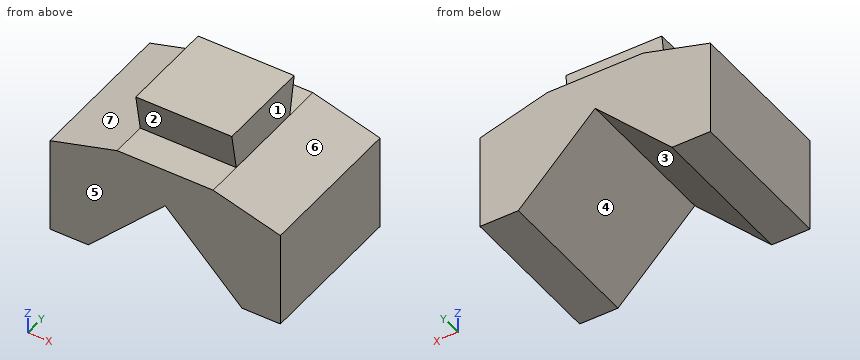
from build123d import *

# Parameters (mm, degrees)
F0_W     = 31.75
F0_H     = 12.7
F1_DEPTH = 25.4
F3_DEPTH = 53.976


with BuildPart() as f1:
    # F0 (on Front) → F1 (new body, symmetric)
    with BuildSketch(Plane.XZ):
        Rectangle(F0_W, F0_H)
        Polygon((15.875, -6.35), (-15.875, -6.35), (-38.1, -12.7), (-38.1, -44.45), (-25.4, -44.45), (0, -19.05), (25.4, -44.45), (38.1, -44.45), (38.1, -12.7), align=None)
    extrude(amount=F1_DEPTH, both=True)

    # F2 (on face) → F3 (cut, through all)
    with BuildSketch(Plane.YZ.offset(15.875)):
        Polygon((-13.635647, -6.35), (-15.875, 6.35), (-25.4, 6.35), (-25.4, -6.35), align=None)
        Polygon((25.4, 6.35), (15.875, 6.35), (13.635647, -6.35), (25.4, -6.35), align=None)
    extrude(amount=-F3_DEPTH, mode=Mode.SUBTRACT)


solid = f1.part
Could you check a few things on this model? Use its own coordinates, in mm. Face numbers are marked on the shaded views. A direction names the side the tool comes from. Give positions to 0.01 mm unless a question says otherwise; leave off trailing zeros. Write each loop counter-clockwise with the first axis right and the second up, starting at its lowest first coordinate (ties: lowest second). Pieces come first, ordered by that corner, then holes. Notation, with made-up numbers: (-22.75, 2.5) -> (-12.75, 2.5) arc R25 ccw to (-12.75, 25.5) -> close; hole circle Ø3 at (-4, 62.5). An arc over 180 degrees is marked (long way). Answer as CSV lines item,"result". Start each with the question number.
(1) If we section it at B-B, the plane x = 8: Write out the boundary of the cut face in (y, z) (3 decimals).
(2) If we section it at D-D, the plane z = -35: Write out the boundary of the cut face in (x, y), and give its area (3 significant figures).
(3) If we mould it in two halves opening along X, with no side actions, what happens to the marked faces 4, 5, 6 and 7? For each: +X half, -X half, draft (parallel to the pull), parting line (faces both ways), or undercut.
(4) Please list where these lines run through material, in increasing order: line 1 (X direction, y = 12, z = -20.5); line 2 (X direction, y = 10, z = -30); line 3 (Z direction, x = 29.5, y = -15).
(5) If we section it at A-A, the plane z = -28.5: Write out the boundary of the cut face in (x, y).
(6) I'm going to push flat-ended pins straight in: pin 1 Ø3 at (x, y) = (17.5, -4) entering from +Z; pin 2 Ø2 at (x, y) = (19, 15) entering from -Z; pin 3 Ø6 at (x, y) = (6.5, 19.5) entering from +Z. Where does each tip first touch, or does it pass through?
(7) If we section it at C-C, the plane y = 0: Write out the boundary of the cut face in (x, z) (3 decimals).
(8) Which directions (+Z, -Z, +X, -X, +Y, -Y) give clear straight access to the entire face, cutting with the end or side of a thin tool? Please do the marked faces 1, 2 and 3.
Answer list:
1,outline,"(-25.4, -27.05) -> (25.4, -27.05) -> (25.4, -6.35) -> (13.636, -6.35) -> (15.875, 6.35) -> (-15.875, 6.35) -> (-13.636, -6.35) -> (-25.4, -6.35) -> close"
2,outline,"(-38.1, -25.4) -> (-15.95, -25.4) -> (-15.95, 25.4) -> (-38.1, 25.4) -> close; (15.95, -25.4) -> (38.1, -25.4) -> (38.1, 25.4) -> (15.95, 25.4) -> close"
2,area,"2,250 mm^2"
3,face 4,"undercut"
3,face 5,"draft"
3,face 6,"+X half"
3,face 7,"-X half"
4,line 1,"-38.1 to -1.45, 1.45 to 38.1"
4,line 2,"-38.1 to -10.95, 10.95 to 38.1"
4,line 3,"-44.45 to -10.24"
5,outline,"(-38.1, -25.4) -> (-9.45, -25.4) -> (-9.45, 25.4) -> (-38.1, 25.4) -> close; (9.45, -25.4) -> (38.1, -25.4) -> (38.1, 25.4) -> (9.45, 25.4) -> close"
6,pin 1,"z = -6.39"
6,pin 2,"z = -39.05"
6,pin 3,"z = -6.35"
7,outline,"(-38.1, -44.45) -> (-25.4, -44.45) -> (0, -19.05) -> (25.4, -44.45) -> (38.1, -44.45) -> (38.1, -12.7) -> (15.875, -6.35) -> (15.875, 6.35) -> (-15.875, 6.35) -> (-15.875, -6.35) -> (-38.1, -12.7) -> close"
8,face 1,"+Z, +X, +Y, -Y"
8,face 2,"+X, -X, -Y"
8,face 3,"-Z, +Y, -Y"
